Could you check a few things on this drawing? It's one solid part, dimensions in mm from its lowest x, y, z. A direction names the side the tool comes from. Coordinates: 2 decimals unless noted, no trailing zeros. Loops run counter-clockwise (first coordinate to the right, second up) from the corner with the lowest first, then second, coordinate; pieces in that order, holes last. Notation, with made-up numbers: M 75.25,1 L 110.25,1 A8 cw 110.25,11 Z; hole C 39.5,36 d8. An arc over 180 degrees is marked long. Answer as a JSON object with one key per item and string values. Group by question number.
Item 1: I'm going to push flat-ended pins straight in: pin 1 Ø6 at (x, y) = (24, 3) entering from +Z; pin 2 Ø2 at (x, z) = (102.5, 15) entering from -Y; pin 3 Ø3 at (x, z) = (15, 4) entering from +Y. Where does each tip first touch, or does it pass through?
Item 2: Which directions (+Z, -Z, +X, -X, +Y, -Y) give clear straight access to the entire face, cutting with the end or side of a thin tool? Please do the marked faces 1, 2 and 3.
Item 3: Suppose I cut it at C-C (x = 37.5). Write out the boundary of the cut face in (y, z).
Item 4: Suppose I cut it at B-B (x = 14). Write out the boundary of the cut face in (y, z), then the cut area to 3 significant figures.
Item 5: Suppose I cut it at D-D (x = 109). Write out the boundary of the cut face in (y, z).
Item 6: Suppose I cut it at A-A (y = 11.5). Write out the boundary of the cut face in (x, z).
Item 7: If I drill on line 1 (Z direction, x = 104, y = 15.5); line 2 (Z direction, x = 88.5, y = 11); line 3 (X direction, y = 20, z = 12.75), over which ranges is the centre line in solid material (lowest first)?
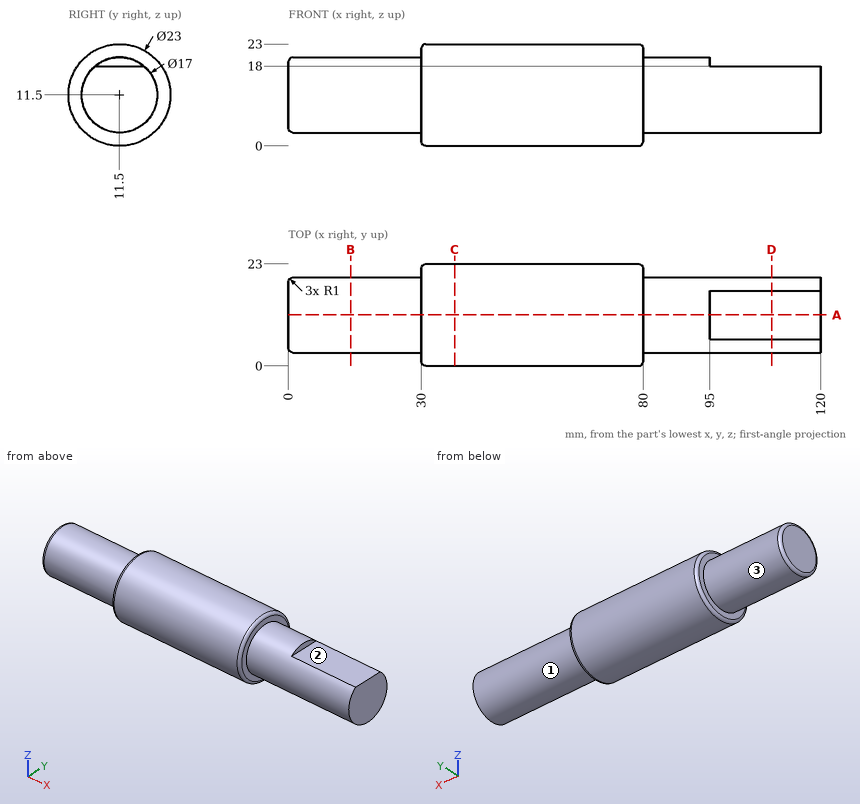
From the geometry:
{
 "1": {"pin 1": "z = 17.98", "pin 2": "y = 3.38", "pin 3": "y = 17.52"},
 "2": {"face 1": "+X", "face 2": "+Z, +X, +Y, -Y", "face 3": "-X"},
 "3": {"outline": "C 11.5,11.5 d23"},
 "4": {"outline": "C 11.5,11.5 d17", "area": "227 mm2"},
 "5": {"outline": "M 6.02,18 A8.5 ccw long 16.98,18 Z"},
 "6": {"outline": "M 0,4 A1 ccw 1,3 L 30,3 L 30,1 A1 ccw 31,0 L 79,0 A1 ccw 80,1 L 80,3 L 120,3 L 120,18 L 95,18 L 95,20 L 80,20 L 80,22 A1 ccw 79,23 L 31,23 A1 ccw 30,22 L 30,20 L 1,20 A1 ccw 0,19 Z"},
 "7": {"line 1": "4 to 18", "line 2": "3.01 to 19.99", "line 3": "30 to 80"}
}
